Part model, mm, in its own coordinate system. A direction names the side the tool comes from. Give positions to 0.01 mm unless a question says otherwise; leave off trailing zeros. Write each loop counter-clockwise with the first axis right and the second up, starting at its lowest first coordinate (ties: lowest second). Pieces come first, ordered by that corner, then holes. Notation, with made-up numbers: M 84.5,17 L 140.5,17 A7 ccw 140.5,23 Z; hole C 72.5,-31.75 d8. An arc over 180 degrees is marked long. Use CSV: the item, a comma, the result in double quotes. Start each with the question number.
1. Mould opens along X. For faces 5 (the face through (-8, 0, 8)), 6 (the face through (21, 0, 0)), 7 (the face through (23, 2, 6)) say: pulls with the +X half, pulls with the -X half, needs draft (parallel to the pull), parting line crosses it, or undercut.
2. Band-saw the part on B-B, the plane x = 29. List the corners of the cut face in (y, z).
3. Band-saw the part on A-A, the plane z = 0. List the corners of the cut face in (x, y).
4. Drop flat-ended pins along their axis: pin 1 Ø8 at (x, y) = (37, 5.5) entering from -Z; pin 2 Ø5.5 at (x, y) = (19.5, -0.5) entering from +Z; pin 3 Ø1.5 at (y, z) = (8.5, -4.5) entering from -X. Give the stop position or say it passes through.
5. Drill centre lines: line 1 along X through (y, z) = (-3.5, 4.05); line 2 along Y through (x, z) = (37, -3.65); line 3 along X through (y, z) = (8.5, -5). Where is each one in solid material? Low to high. Write a range as from..to.
6. Band-saw the part on C-C, the plane y = 8.5. List the corners of the cut face in (x, z), then the cut area to 3 significant figures.
7. 3-axis set-ups, long thin cutter, end or side, ignore diameter. For faces 1 (the face through (-14, 1, 0)), 2 (the face through (21, 10, -3)), 3 (the face through (23, 2, -6)), 4 (the face through (-9, -2.5, 0)): which of +Z, -Z, +X, -X, +Y, -Y reach the whole face in a straight line?
8. Band-saw the part on D-D, the plane y = -3.5. Count the separate pieces of the cut face and the enclosed holes in it, then the cut area to 3 significant figures.
from build123d import *

# Parameters (mm, degrees)
BOSS_EXTRUDE1_DEPTH     = 7.5
SKETCH4_R               = 4.1
CUT_EXTRUDE1_DEPTH      = 10
SKETCH5_R               = 1.5
CUT_EXTRUDE2_DEPTH      = 5
CUT_EXTRUDE4_REACH      = 40.591
CUT_EXTRUDE4_END_RADIUS = 4.1
SKETCH7_R               = 1.5
BOSS_EXTRUDE2_DEPTH     = 20
SKETCH10_W              = 20
SKETCH10_H              = 3
CUT_EXTRUDE5_DEPTH      = 20
CUT_EXTRUDE6_DEPTH      = 46.249309387
CUT_EXTRUDE6_DEPTH_BACK = 46.249309387
SKETCH11_R              = 1.5


with BuildPart() as part:
    # Sketch2 → Boss-Extrude1 (new, symmetric)
    with BuildSketch(Plane(origin=(0, 0, 0), x_dir=(1, 0, 0), z_dir=(0, 1, 0))):
        Polygon((-16, -8), (-16, 8), (0, 8), (16, 5.5), (21, 5.5), (21, -5.5), (16, -5.5), (0, -8), align=None)
    extrude(amount=BOSS_EXTRUDE1_DEPTH, both=True)

    # Sketch4 → Cut-Extrude1 (cut)
    with BuildSketch(Plane(origin=(0, 7.5, 0), x_dir=(1, 0, 0), z_dir=(0, 1, 0))):
        with Locations(Location((-7.259972257, 0, 0), (0, 0, 270))):
            Circle(SKETCH4_R)
    extrude(amount=-CUT_EXTRUDE1_DEPTH, mode=Mode.SUBTRACT)

    # Sketch5 → Cut-Extrude2 (cut)
    with BuildSketch(Plane(origin=(0, -2.5, 0), x_dir=(1, 0, 0), z_dir=(0, 1, 0))):
        with Locations(Location((-7.259972257, 0, 0), (0, 0, 270))):
            Circle(SKETCH5_R)
    extrude(amount=-CUT_EXTRUDE2_DEPTH, mode=Mode.SUBTRACT)

    # Cut-Extrude4: up to this cylinder (the profile starts outside it)
    cut_extrude4_end = Plane(origin=(-7.259972257, 2.5, 0), z_dir=(0, 1, 0)) * Cylinder(CUT_EXTRUDE4_END_RADIUS, 90.382, mode=Mode.PRIVATE)
    # Sketch7 → Cut-Extrude4 (cut, up to the surface)
    with BuildSketch(Plane.ZY.offset(16), mode=Mode.PRIVATE) as cut_extrude4_sk1:
        with Locations((0, 2.5)):
            Circle(SKETCH7_R)
    cut_extrude4_tool1 = extrude(cut_extrude4_sk1.sketch, amount=-CUT_EXTRUDE4_REACH, mode=Mode.PRIVATE) - cut_extrude4_end
    add(cut_extrude4_tool1.solids().sort_by_distance((-16, 2.5, 0))[0], mode=Mode.SUBTRACT)

    # Sketch9 → Boss-Extrude2 (add)
    with BuildSketch(Plane(origin=(0, -7.5, 0), x_dir=(1, 0, 0), z_dir=(0, 1, 0))):
        Polygon((21, 5.5), (25, 6.5), (41, 6.5), (41, -6.5), (25, -6.5), (21, -5.5), align=None)
    extrude(amount=BOSS_EXTRUDE2_DEPTH)

    # Sketch10 → Cut-Extrude5 (cut)
    with BuildSketch(Plane(origin=(0, 12.5, 0), x_dir=(1, 0, 0), z_dir=(0, 1, 0))):
        with Locations((31, 0)):
            Rectangle(SKETCH10_W, SKETCH10_H)
    extrude(amount=-CUT_EXTRUDE5_DEPTH, mode=Mode.SUBTRACT)

    # Sketch11 → Cut-Extrude6 (cut, two sides: drawn at the far end of the back side and taken through both)
    with BuildSketch(Plane(origin=(0, 0, -6.5), x_dir=(-1, 0, 0), z_dir=(0, 0, -1)).offset(-CUT_EXTRUDE6_DEPTH_BACK)):
        with Locations((-37, 8.5)):
            Circle(SKETCH11_R)
        with Locations((-29, 8.5)):
            Circle(SKETCH11_R)
        with Locations((-37, -3.5)):
            Circle(SKETCH11_R)
        with Locations((-29, -3.5)):
            Circle(SKETCH11_R)
    extrude(amount=CUT_EXTRUDE6_DEPTH + CUT_EXTRUDE6_DEPTH_BACK, mode=Mode.SUBTRACT)


solid = part.part
Output:
1,face 5,"needs draft"
1,face 6,"pulls with the +X half"
1,face 7,"undercut"
2,outline,"M -7.5,-6.5 L -5,-6.5 L -5,-1.5 L -7.5,-1.5 Z; M -7.5,1.5 L -5,1.5 L -5,6.5 L -7.5,6.5 Z; M -2,-6.5 L 7,-6.5 L 7,-1.5 L -2,-1.5 Z; M -2,1.5 L 7,1.5 L 7,6.5 L -2,6.5 Z; M 10,-6.5 L 12.5,-6.5 L 12.5,-1.5 L 10,-1.5 Z; M 10,1.5 L 12.5,1.5 L 12.5,6.5 L 10,6.5 Z"
3,outline,"M -16,-7.5 L -8.76,-7.5 L -8.76,-2.5 L -11.36,-2.5 L -11.36,1 L -16,1 Z; M -16,4 L -11.36,4 L -11.36,7.5 L -16,7.5 Z; M -5.76,-7.5 L 21,-7.5 L 21,7.5 L -3.16,7.5 L -3.16,-2.5 L -5.76,-2.5 Z"
4,pin 1,"stops at z = -6.5"
4,pin 2,"stops at z = 5.81"
4,pin 3,"stops at x = 21"
5,line 1,"x = -16..27.5, 30.5..35.5, 38.5..41"
5,line 2,"y = -7.5..-5, -2..7, 10..12.5"
5,line 3,"x = 21..27.5, 30.5..35.5, 38.5..41"
6,outline,"M 21,-5.5 L 25,-6.5 L 27.5,-6.5 L 27.5,-1.5 L 21,-1.5 Z; M 21,1.5 L 27.5,1.5 L 27.5,6.5 L 25,6.5 L 21,5.5 Z; M 30.5,-6.5 L 35.5,-6.5 L 35.5,-1.5 L 30.5,-1.5 Z; M 30.5,1.5 L 35.5,1.5 L 35.5,6.5 L 30.5,6.5 Z; M 38.5,-6.5 L 41,-6.5 L 41,-1.5 L 38.5,-1.5 Z; M 38.5,1.5 L 41,1.5 L 41,6.5 L 38.5,6.5 Z"
6,area,"136 mm²"
7,face 1,"-X"
7,face 2,"+Z, -Z, -X, +Y"
7,face 3,"-Z, +Y, -Y"
7,face 4,"+Y"
8,separate pieces,"5"
8,enclosed holes,"1"
8,area,"656 mm²"
